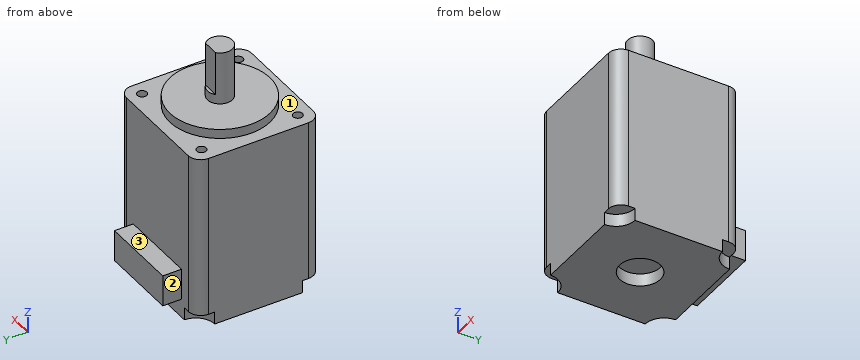
from build123d import *

# Parameters (mm, degrees)
ESBO_O1_W                = 20
ESBO_O1_H                = 20
RESSALTO_EXTRUS_O1_DEPTH = 28
ESBO_O2_R                = 3.25
ESBO_O2_R_2              = 3
CORTE_EXTRUS_O1_DEPTH    = 2
ESBO_O3_W                = 12.5
ESBO_O3_H                = 5
RESSALTO_EXTRUS_O2_DEPTH = 3
FILETE1_R                = 2
ESBO_O4_R                = 8
RESSALTO_EXTRUS_O3_DEPTH = 1.5
ESBO_O5_R                = 2
RESSALTO_EXTRUS_O4_DEPTH = 8.5
ESBO_O6_W                = 5.42124419
ESBO_O6_H                = 2.409441862
CORTE_EXTRUS_O2_DEPTH    = 7
ESBO_O7_R                = 0.75
CORTE_EXTRUS_O3_DEPTH    = 5


with BuildPart() as part:
    # Esboço1 → Ressalto-extrusão1 (new body)
    with BuildSketch(Plane.XY):
        Rectangle(ESBO_O1_W, ESBO_O1_H)
    extrude(amount=RESSALTO_EXTRUS_O1_DEPTH)

    # Esboço2 → Corte-extrusão1 (cut)
    with BuildSketch(Plane(origin=(0, 0, 0), x_dir=(-1, 0, 0), z_dir=(0, 0, -1))):
        Circle(ESBO_O2_R)
        with Locations((-10, 10)):
            Circle(ESBO_O2_R_2)
        with Locations((10, 10)):
            Circle(ESBO_O2_R_2)
        with Locations((10, -10)):
            Circle(ESBO_O2_R_2)
        with Locations((-10, -10)):
            Circle(ESBO_O2_R_2)
    extrude(amount=-CORTE_EXTRUS_O1_DEPTH, mode=Mode.SUBTRACT)

    # Esboço3 → Ressalto-extrusão2 (add)
    with BuildSketch(Plane(origin=(0, 10, 0), x_dir=(1, 0, 0), z_dir=(0, 1, 0))):
        with Locations((0, -5.5)):
            Rectangle(ESBO_O3_W, ESBO_O3_H)
    extrude(amount=RESSALTO_EXTRUS_O2_DEPTH)

    # Filete1
    filete1_edges = [part.edges().sort_by_distance(p)[0] for p in [
        (10, -10, 15),
        (-10, -10, 15),
        (-10, 10, 15),
        (10, 10, 15),
    ]]
    fillet(filete1_edges, radius=FILETE1_R)

    # Esboço4 → Ressalto-extrusão3 (add)
    with BuildSketch(Plane.XY.offset(28)):
        Circle(ESBO_O4_R)
    extrude(amount=RESSALTO_EXTRUS_O3_DEPTH)

    # Esboço5 → Ressalto-extrusão4 (add)
    with BuildSketch(Plane.XY.offset(29.5)):
        Circle(ESBO_O5_R)
    extrude(amount=RESSALTO_EXTRUS_O4_DEPTH)

    # Esboço6 → Corte-extrusão2 (cut)
    with BuildSketch(Plane.XY.offset(38)):
        with Locations((0, 2.704720931)):
            Rectangle(ESBO_O6_W, ESBO_O6_H)
    extrude(amount=-CORTE_EXTRUS_O2_DEPTH, mode=Mode.SUBTRACT)

    # Esboço7 → Corte-extrusão3 (cut)
    with BuildSketch(Plane.XY.offset(28)):
        with Locations((-7.7, 7.7)):
            Circle(ESBO_O7_R)
        with Locations((7.7, 7.7)):
            Circle(ESBO_O7_R)
        with Locations((7.7, -7.7)):
            Circle(ESBO_O7_R)
        with Locations((-7.7, -7.7)):
            Circle(ESBO_O7_R)
    extrude(amount=-CORTE_EXTRUS_O3_DEPTH, mode=Mode.SUBTRACT)


solid = part.part
Geometry: final body of the model. Coordinates: model frame, mm. Face numbers are marked on the shaded views. A direction names the side the tool comes from. Round coordinates to 2 decimals unless told otherwise and drop trailing zeros. Order: outer loops, then holes, each group sorted by start corner. A loop starts at its lowest first (then second) coordinate and runs counter-clockwise, first axis right, second up.
Q1. Section D-D, the plane x = 0. Output: boundary loops of the cut face in (y, z).
Result sheet:
outline: (-10, 0) - (-3.25, 0) - (-3.25, 2) - (3.25, 2) - (3.25, 0) - (10, 0) - (10, 3) - (13, 3) - (13, 8) - (10, 8) - (10, 28) - (8, 28) - (8, 29.5) - (2, 29.5) - (2, 31) - (1.5, 31) - (1.5, 38) - (-2, 38) - (-2, 29.5) - (-8, 29.5) - (-8, 28) - (-10, 28) - close
Q2. Pin query (flat end, axial travel): pin 1 (1 mm diameter, centred on x = 6.5, y = -7, fed in from -Z); pin 2 (0.7 mm diameter, centred on x = 7.5, y = 8, fed in from +Z); pin 3 (2 mm diameter, centred on x = 1, y = -1.5, fed in from -Z); pin 4 (1.5 mm diameter, centred on y = 11, z = 4.5, fed in from +X). Return the tip coordinate at first contact, or that it passes through.
Result sheet:
pin 1: stops at z = 0
pin 2: stops at z = 23
pin 3: stops at z = 2
pin 4: stops at x = 6.25
Q3. Section C-C, the plane z = 22.5. Output: boundary loops of the cut face in (x, y).
Result sheet:
outline: (-10, -8) arc R2 ccw to (-8, -10) - (8, -10) arc R2 ccw to (10, -8) - (10, 8) arc R2 ccw to (8, 10) - (-8, 10) arc R2 ccw to (-10, 8) - close
Q4. Material intervals for probe 1 along Y at (x, z) = (-7.7, 24.2); probe 2 along Y at (x, z) = (0, 1.4); probe 3 along Y at (x, z) = (1.25, 23), sorted ascending.
Result sheet:
probe 1: y = -10 to -8.45, -6.95 to 6.95, 8.45 to 10
probe 2: y = -10 to -3.25, 3.25 to 10
probe 3: y = -10 to 10
Q5. Access query for the marked faces 1, 2 and 3. Directions: +Z, -Z, +X, -X, +Y, -Y. A direction counts if a zero-diameter tool reaches every point of the face in a straight line with its end or side. Return the directions, or none.
Result sheet:
face 1: +Z
face 2: +Z, -Z, -X, +Y
face 3: +Z, +X, -X, +Y
Q6. Section A-A, the plane z = 27. Output: boundary loops of the cut face in (x, y), and give its area (3 significant figures).
Result sheet:
outline: (-10, -8) arc R2 ccw to (-8, -10) - (8, -10) arc R2 ccw to (10, -8) - (10, 8) arc R2 ccw to (8, 10) - (-8, 10) arc R2 ccw to (-10, 8) - close; hole circle Ø1.5 at (-7.7, -7.7); hole circle Ø1.5 at (-7.7, 7.7); hole circle Ø1.5 at (7.7, -7.7); hole circle Ø1.5 at (7.7, 7.7)
area: 389 mm2
Q7. Section B-B, the plane y = 0. Output: boundary loops of the cut face in (x, z).
Result sheet:
outline: (-10, 0) - (-3.25, 0) - (-3.25, 2) - (3.25, 2) - (3.25, 0) - (10, 0) - (10, 28) - (8, 28) - (8, 29.5) - (2, 29.5) - (2, 38) - (-2, 38) - (-2, 29.5) - (-8, 29.5) - (-8, 28) - (-10, 28) - close
